Build history of the part. All positions in model axes, mm. A direction names the side the tool comes from. Give positions to 0.01 mm unless a question says otherwise; leave off trailing zeros. Loops run counter-clockwise (first coordinate to the right, second up) from the corner with the lowest first, then second, coordinate; pieces in that order, holes last. Notation, with made-up numbers: (1.5, -9.75) -> (38.5, -9.75) arc R30 cw to (38.5, 20.25) -> close; hole circle Ø2 at (74.25, 51). An arc over 180 degrees is marked (long way). Answer as a JSON object with one key per item and string values. Group by question number.
Q1. Band-saw the part on B-B, the plane x = -38.1. Write the cut outline in (y, z), plus the area to 3 significant figures.
Q2. Band-saw the part on A-A, the plane y = -12.5. Write the cut outline in (x, z) (3 decimals).
Q3. Tool access for faces 1 (the flat face through (47.625, -22, 3)), 2 (the flat face through (34.836, -29, 3)): list every direction of +Z, -Z, +X, -X, +Y, -Y with a clear straight run to the whole face (end or side of a thin tool).
Q4. Band-saw the part on C-C, the plane z = 1.5. Count the separate pieces of the cut face and the enclosed holes in it, plus the area to 3 significant figures.
Q5. Two-plate mould, pull along X, no slides. Class faces 3 (the cylindrical face through (38.172, -35.013, 3.131)), 4 (the cylindrical face through (-14.274, 0.628, 3.131)), 5 (the flat face through (29.57, 5.39, 3.13)), 6 (the flat face through (-1, -38.1, 3)): pulls with the +X half, pulls with the -X half, needs draft (parallel to the pull), parting line crosses it, or undercut.
Q6. Band-saw the part on D-D, the plane y = -33. Write the cut outline in (x, z) (3 decimals).
Q7. Drop a flat-ended pin along its axis: pin 1 (10 mm diameter, centred on x = 30.5, y = -5, fed in from -Z). Give the stop position or say it passes through.
Q8. Wall check: probe 1 along Y at (x, z) = (0, 4); probe 2 along X at (y, z) = (1, 4); probe 3 along X at (y, z) = (-0.5, 2). Give the ranges that are in metal, low to high. Write a range as from..to.
from build123d import *

# Parameters (mm, degrees)
SKETCH1_R           = 14.2875
BOSS_EXTRUDE1_DEPTH = 6.35
FILLET1_R           = 0.508


with BuildPart() as part:
    # Sketch1 → Boss-Extrude1 (new body)
    with BuildSketch(Plane.XY):
        with BuildLine():
            Line((-11.249807725, 17.301682936), (-47.625, -6.35))
            Line((-47.625, -6.35), (-47.625, -38.1))
            Line((-47.625, -38.1), (47.625, -38.1))
            Line((47.625, -38.1), (47.625, -6.35))
            Line((47.625, -6.35), (11.249807725, 17.301682936))
            ThreePointArc((11.249807725, 17.301682936), (0, 20.6375), (-11.249807725, 17.301682936))
        make_face()
        Circle(SKETCH1_R, mode=Mode.SUBTRACT)
        with BuildLine():
            Line((-34.8361, -25.4), (-34.8361, -31.75))
            ThreePointArc((-34.8361, -31.75), (-38.1, -35.0139), (-41.3639, -31.75))
            Line((-41.3639, -31.75), (-41.3639, -25.4))
            ThreePointArc((-41.3639, -25.4), (-38.1, -22.1361), (-34.8361, -25.4))
        make_face(mode=Mode.SUBTRACT)
        with BuildLine():
            Line((41.3639, -25.4), (41.3639, -31.75))
            ThreePointArc((41.3639, -31.75), (38.1, -35.0139), (34.8361, -31.75))
            Line((34.8361, -31.75), (34.8361, -25.4))
            ThreePointArc((34.8361, -25.4), (38.1, -22.1361), (41.3639, -25.4))
        make_face(mode=Mode.SUBTRACT)
    extrude(amount=BOSS_EXTRUDE1_DEPTH)

    # Fillet1
    fillet1_edges = [part.edges().sort_by_distance(p)[0] for p in [
        (47.625, -6.35, 3.175),
        (47.625, -38.1, 3.175),
        (-47.625, -38.1, 3.175),
        (-47.625, -6.35, 3.175),
    ]]
    fillet(fillet1_edges, radius=FILLET1_R)


solid = part.part
Worked answers:
{
 "1": {"outline": "(-38.1, 0) -> (-35.01, 0) -> (-35.01, 6.35) -> (-38.1, 6.35) -> close; (-22.14, 0) -> (-0.16, 0) -> (-0.16, 6.35) -> (-22.14, 6.35) -> close", "area": "159 mm2"},
 "2": {"outline": "(-47.625, 0) -> (-6.92, 0) -> (-6.92, 6.35) -> (-47.625, 6.35) -> close; (6.92, 0) -> (47.625, 0) -> (47.625, 6.35) -> (6.92, 6.35) -> close"},
 "3": {"face 1": "+Z, -Z, +X, +Y, -Y", "face 2": "+Z, -Z"},
 "4": {"separate pieces": "1", "enclosed holes": "3", "area": "3,680 mm2"},
 "5": {"face 3": "undercut", "face 4": "undercut", "face 5": "pulls with the +X half", "face 6": "needs draft"},
 "6": {"outline": "(-47.625, 0) -> (-41.115, 0) -> (-41.115, 6.35) -> (-47.625, 6.35) -> close; (-35.085, 0) -> (35.085, 0) -> (35.085, 6.35) -> (-35.085, 6.35) -> close; (41.115, 0) -> (47.625, 0) -> (47.625, 6.35) -> (41.115, 6.35) -> close"},
 "7": {"pin 1": "z = 0"},
 "8": {"probe 1": "-38.1..-14.29, 14.29..20.64", "probe 2": "-36.32..-14.25, 14.25..36.32", "probe 3": "-38.63..-14.28, 14.28..38.63"}
}
